from build123d import *

# Parameters (mm, degrees)
SKETCH_2_R          = 5.9
EXTRUDE_1_DEPTH     = 11
SKETCH_3_R          = 7.15
EXTRUDE_2_DEPTH     = 1
SKETCH_4_R          = 3.1
SKETCH_4_R_2        = 0.5
CUT_EXTRUDE_1_DEPTH = 5
FILLET_1_R          = 0.3
FILLET_2_R          = 0.3
SKETCH_5_W          = 16.4
SKETCH_5_H          = 21
SKETCH_5_W_2        = 10.4
SKETCH_5_H_2        = 15
CUT_EXTRUDE_2_DEPTH = 11
SKETCH_6_W          = 2.420538387
SKETCH_6_H          = 0.443765371
SKETCH_6_W_2        = 2.501222999
SKETCH_6_H_2        = 0.56479229
SKETCH_6_W_3        = 0.524449984
SKETCH_6_H_3        = 2.38019608
EXTRUDE_3_DEPTH     = 5
FILLET_3_R          = 1
EXTRUDE_START       = -4
EXTRUDE_4_DEPTH     = 1.5


with BuildPart() as part:
    # 草图2 → 凸台-拉伸1 (new body)
    with BuildSketch(Plane(origin=(0, 0, 0), x_dir=(1, 0, 0), z_dir=(0, 1, 0))):
        with Locations(Location((0, 0, 0), (0, 0, 270))):
            Circle(SKETCH_2_R)
    extrude(amount=EXTRUDE_1_DEPTH)

    # 草图3 → 凸台-拉伸2 (add)
    with BuildSketch(Plane.XZ):
        with Locations(Location((0, 0, 0), (0, 0, 270))):
            Circle(SKETCH_3_R)
    extrude(amount=EXTRUDE_2_DEPTH)

    # 草图4 → 切除-拉伸1 (cut)
    with BuildSketch(Plane.XZ.offset(1)):
        with Locations(Location((0, 2.5, 0), (0, 0, 270))):
            Circle(SKETCH_4_R)
        with Locations(Location((0, 2.5, 0), (0, 0, 270))):
            Circle(SKETCH_4_R_2, mode=Mode.SUBTRACT)
    extrude(amount=-CUT_EXTRUDE_1_DEPTH, mode=Mode.SUBTRACT)

    # 圆角1
    fillet_1_edges = [part.edges().sort_by_distance(p)[0] for p in [
        (0, -1, 3),
    ]]
    fillet(fillet_1_edges, radius=FILLET_1_R)

    # 圆角2
    fillet_2_edges = [part.edges().sort_by_distance(p)[0] for p in [
        (0, -1, 7.15),
    ]]
    fillet(fillet_2_edges, radius=FILLET_2_R)

    # 草图5 → 切除-拉伸2 (cut)
    with BuildSketch(Plane(origin=(0, 11, 0), x_dir=(1, 0, 0), z_dir=(0, 1, 0))):
        Rectangle(SKETCH_5_W, SKETCH_5_H)
        Rectangle(SKETCH_5_W_2, SKETCH_5_H_2, mode=Mode.SUBTRACT)
    extrude(amount=-CUT_EXTRUDE_2_DEPTH, mode=Mode.SUBTRACT)

    # 草图6 → 凸台-拉伸3 (add)
    with BuildSketch(Plane(origin=(0, 11, 0), x_dir=(1, 0, 0), z_dir=(0, 1, 0))):
        with Locations((-1.331296113, 3.842604689)):
            Rectangle(SKETCH_6_W, SKETCH_6_H)
        with Locations((2.38019608, 2.531479729)):
            Rectangle(SKETCH_6_W_2, SKETCH_6_H_2)
        with Locations((-3.227384515, -1.906173979)):
            Rectangle(SKETCH_6_W_3, SKETCH_6_H_3)
    extrude(amount=EXTRUDE_3_DEPTH)

    # 圆角3
    fillet_3_edges = [part.edges().sort_by_distance(p)[0] for p in [
        (-0.121026919, 16, -3.842604688),
        (-2.541565306, 16, -3.842604688),
        (3.630807579, 16, -2.531479729),
        (1.12958458, 16, -2.531479729),
        (-3.227384515, 16, 0.716075939),
        (-3.227384515, 16, 3.096272019),
    ]]
    fillet(fillet_3_edges, radius=FILLET_3_R)

    # 草图7 → 凸台-拉伸4 (add)
    with BuildSketch(Plane(origin=(0, 11, 0), x_dir=(1, 0, 0), z_dir=(0, 1, 0)).offset(EXTRUDE_START)):
        Polygon((-3.406366588, 5.9), (-6.812733176, 0), (-3.406366588, -5.9), (3.406366588, -5.9), (6.812733176, 0), (3.406366588, 5.9), align=None)
    extrude(amount=-EXTRUDE_4_DEPTH)

    # 草图8 → 切除-旋转1 (revolve, cut)
    with BuildSketch(Plane.XY, mode=Mode.PRIVATE) as cut_revolve_1_sk:
        Polygon((-6.812733176, 7), (-6.812733176, 6.5), (-5.2, 7), align=None)
        Polygon((-5.2, 5.5), (-6.812733176, 5.5), (-6.812733176, 6), align=None)
    revolve(cut_revolve_1_sk.sketch.rotate(Axis((0, 11, 0), (0, -1, 0)), 180.000000014), axis=Axis((0, 11, 0), (0, -1, 0)), mode=Mode.SUBTRACT)


solid = part.part
Verification items for the finished model (mm, model axes). A direction names the side the tool comes from. Coordinates: 2 decimals unless noted, no trailing zeros. Write each loop counter-clockwise with the first axis right and the second up, starting at its lowest first coordinate (ties: lowest second). Pieces come first, ordered by that corner, then holes. Notation, with made-up numbers: M -39,-26.75 L 19,-26.75 A24 ccw 19,-14.75 Z; hole C 20,-2 d8. An arc over 180 degrees is marked long. Use a Markdown table: item, result.
Q1. Set-up check for faces 1 (the face through (-5.086, 6.257, -2.991)), 2 (the face through (-2.965, 13, 2)), 3 (the face through (-0.1, 9, 5.9)): record each of +Z, -Z, +X, -X, +Y, -Y from which the full face is reachable in a straight line by a thin tool's end or side.
Reply:
| item | result |
|---|---|
| face 1 | -Z, -X, +Y |
| face 2 | +Z, -Z, +X, +Y |
| face 3 | +Z, +Y |
Q2. Thickness scan on line 1 (X direction, y = 2.8, z = 2.5); line 2 (Y direction, x = -5, z = 3); line 3 (Y direction, x = -0.5, z = -2.5). Record the ranges inside material, lowest first.
Reply:
| item | result |
|---|---|
| line 1 | x = -5.2 to -3.1, -0.5 to 0.5, 3.1 to 5.2 |
| line 2 | y = -1 to 5.5, 5.7 to 6.8, 7 to 11 |
| line 3 | y = -1 to 11 |
Q3. Sectioned sample at A-A, the plane y = 2.25. Record the boundary of the cut face in (x, z).
Reply:
| item | result |
|---|---|
| outline | M -5.2,-2.79 A5.9 ccw 5.2,-2.79 L 5.2,2.79 A5.9 ccw -5.2,2.79 Z; C 0,2.5 d1; hole C 0,2.5 d6.2 |
Q4. Go/stop test with flat-tipped pins: P1, Ø4.5, axis at y = 9.5, z = -0.5, coming from the -X side; P2, Ø2.5, axis at x = -1, y = 14.5, coming from the -Z side; P3, Ø6.5, axis at x = 1, z = 3, coming from the -Y side; P4, Ø2.5, axis at y = 13, z = 2.5, coming from the -X side. Record where each tip stops, or that it passes through.
Reply:
| item | result |
|---|---|
| P1 | stops at x = -5.2 |
| P2 | stops at z = -4.06 |
| P3 | stops at y = -1 |
| P4 | stops at x = -3.49 |
Q5. Draft check along Y on faces 4 (the face through (0.1, 2.7, -5.9)), 5 (the face through (5.086, 6.257, 2.991)), 6 (the face through (1.415, 15.699, -2.535)), 7 (the face through (-1, 4, 3)). Enter one of: +Y half, -Y half, draft (parallel to the pull), parting line (faces both ways), or undercut.
Reply:
| item | result |
|---|---|
| face 4 | undercut |
| face 5 | draft |
| face 6 | +Y half |
| face 7 | -Y half |
Q6. Sectioned sample at B-B, the plane y = 13. Record the boundary of the cut face in (x, z), plus the area to 3 significant figures.
Reply:
| item | result |
|---|---|
| outline | M -3.49,0.72 L -2.97,0.72 L -2.97,3.1 L -3.49,3.1 Z; M -2.54,-4.06 L -0.12,-4.06 L -0.12,-3.62 L -2.54,-3.62 Z; M 1.13,-2.81 L 3.63,-2.81 L 3.63,-2.25 L 1.13,-2.25 Z |
| area | 3.74 mm² |
